Here's how the part is built. I have some questions about the finished solid (model axes, mm). A direction names the side the tool comes from. Coordinates: 2 decimals unless noted, no trailing zeros. Write each loop counter-clockwise with the first axis right and the second up, starting at its lowest first coordinate (ties: lowest second). Pieces come first, ordered by that corner, then holes. Notation, with made-up numbers: (38, 48.5) -> (80, 48.5) arc R21 ccw to (80, 87.5) -> close; hole circle Ø3 at (-4, -35.5). An arc over 180 degrees is marked (long way). Put each result on its own line as item: value.
Autodesk Inventor part; units mm, degrees
ref_plane "YZ Plane" through (0, 0, 0) normal (1, 0, 0) x (0, 1, 0)
ref_plane "XZ Plane" through (0, 0, 0) normal (0, 1, 0) x (-1, 0, 0)
ref_plane "XY Plane" through (0, 0, 0) normal (0, 0, 1) x (1, 0, 0)
sketch "Sketch1" plane through (0, 0, 0) normal (0, 1, 0) x (-1, 0, 0)
  line L0 (0, 0) -> (128, 0)
  line L1 (128, 0) -> (128, 22)
  line L2 (52, 14) -> (52, 8)
  line L3 (52, 8) -> (22, 8)
  line L4 (22, 8) -> (22, 14)
  circle A0 centre (5.5, 18.5) radius 2.25
  circle A1 centre (5.5, 18.5) radius 4.5 construction
  circle A2 centre (25.5, 18.5) radius 2.25
  circle A3 centre (25.5, 18.5) radius 4.5 construction
  line L5 (33, 14) -> (44, 14) construction
  circle A4 centre (38.5, 19.099) radius 7.5 construction
  circle A5 centre (38.5, 19.099) radius 4 construction
  line L6 (33, 23) -> (33, 14)
  line L7 (44, 14) -> (44, 23)
  line L8 (22, 14) -> (33, 14)
  line L9 (44, 14) -> (52, 14)
  line L10 (0, 14) -> (4, 14)
  line L11 (4, 14) -> (4, 8)
  line L12 (4, 8) -> (0, 8)
  line L13 (0, 23) -> (0, 14)
  line L14 (0, 8) -> (0, 0)
  line L15 (11.5, 23) -> (11.5, 29)
  line L16 (13.5, 31) -> (17.5, 31)
  line L17 (19.5, 29) -> (19.5, 23)
  arc A6 (13.5, 31) -> (11.5, 29) centre (13.5, 29) ccw
  arc A7 (19.5, 29) -> (17.5, 31) centre (17.5, 29) ccw
  line L18 (33, 23) -> (19.5, 23)
  line L19 (11.5, 23) -> (0, 23)
  line L20 (50, 23) -> (50, 29)
  line L21 (52, 31) -> (56, 31)
  line L22 (58, 29) -> (58, 23)
  arc A8 (52, 31) -> (50, 29) centre (52, 29) ccw
  arc A9 (58, 29) -> (56, 31) centre (56, 29) ccw
  line L23 (68, 23) -> (58, 23)
  line L24 (50, 23) -> (44, 23)
  line L25 (68, 23) -> (68, 22)
  line L26 (68, 22) -> (128, 22)
  line L27 (19.5, 16.7896) -> (15.5, 14.4802)
  line L28 (15.5, 14.4802) -> (11.5, 16.7896)
  line L29 (11.5, 16.7896) -> (11.5, 21.4084)
  line L30 (11.5, 21.4084) -> (15.5, 23.7178)
  line L31 (15.5, 23.7178) -> (19.5, 21.4084)
  line L32 (19.5, 21.4084) -> (19.5, 16.7896)
  point P0 (15.5, 19.099)
  point P1 (0, 18.5)
  point P2 (15.5, 31)
  point P3 (15.5, 19.099)
  dimension "d0" = 6
  dimension "d1" = 8
  dimension "d3" = 4.5
  dimension "d4" = 9
  dimension "d5" = 4.5
  dimension "d6" = 9
  dimension "d8" = 11
  dimension "d9" = 8
  dimension "d10" = 15
  dimension "d11" = 9
  dimension "d12" = 4
  dimension "d13" = 5.5
  dimension "d14" = 10
  dimension "d15" = 10
  dimension "d16" = 2
  dimension "d17" = 8
  dimension "d18" = 8
  dimension "d19" = 23
  dimension "d20" = 30
  dimension "d21" = 18
  dimension "d23" = 2
  dimension "d24" = 8
  dimension "d25" = 6
  dimension "d26" = 8
  dimension "d27" = 10
  dimension "d29" = 60
  dimension "d30" = 8
extrude "Extrusion1" add sketch "Sketch1" along normal blind 6
sketch "Sketch2" plane through (0, 6, 0) normal (0, 1, 0) x (1, 0, 0)
  line L0 (-128, 0) -> (-128, -22)
  line L1 (-128, -22) -> (-68, -22)
  line L2 (-68, -22) -> (-68, -23)
  line L3 (-120, -22) -> (-112, -22)
  line L4 (-112, -22) -> (-112, -26)
  line L5 (-114, -28) -> (-118, -28)
  line L6 (-120, -26) -> (-120, -22)
  line L7 (-84, -22) -> (-76, -22)
  line L8 (-76, -22) -> (-76, -26)
  line L9 (-78, -28) -> (-82, -28)
  line L10 (-84, -26) -> (-84, -22)
  arc A0 (-84, -26) -> (-82, -28) centre (-82, -26) ccw
  arc A1 (-78, -28) -> (-76, -26) centre (-78, -26) ccw
  arc A2 (-114, -28) -> (-112, -26) centre (-114, -26) ccw
  arc A3 (-120, -26) -> (-118, -28) centre (-118, -26) ccw
  dimension "d33" = 2
  dimension "d34" = 8
  dimension "d35" = 6
  dimension "d36" = 8
  dimension "d37" = 8
  dimension "d38" = 8
extrude "Extrusion2" add sketch "Sketch2" against normal blind 6
sketch "Sketch3" plane through (0, 6, 0) normal (0, 1, 0) x (1, 0, 0)
  line L0 (0, 0) -> (-128, 0)
  line L1 (-112, -26) -> (-112, -22)
  line L2 (-76, -26) -> (-76, -22)
  line L3 (0, -8) -> (0, 0)
  line L4 (-120, 0) -> (-112, 0)
  line L5 (-112, 0) -> (-112, 4)
  line L6 (-114, 6) -> (-118, 6)
  line L7 (-120, 4) -> (-120, 0)
  line L8 (-84, 0) -> (-76, 0)
  line L9 (-76, 0) -> (-76, 4)
  line L10 (-78, 6) -> (-82, 6)
  line L11 (-84, 4) -> (-84, 0)
  line L12 (-63, 0) -> (-55, 0)
  line L13 (-55, 0) -> (-55, 4)
  line L14 (-57, 6) -> (-61, 6)
  line L15 (-63, 4) -> (-63, 0)
  line L16 (-12, 0) -> (-4, 0)
  line L17 (-4, 0) -> (-4, 4)
  line L18 (-6, 6) -> (-10, 6)
  line L19 (-12, 4) -> (-12, 0)
  arc A0 (-118, 6) -> (-120, 4) centre (-118, 4) ccw
  arc A1 (-112, 4) -> (-114, 6) centre (-114, 4) ccw
  arc A2 (-82, 6) -> (-84, 4) centre (-82, 4) ccw
  arc A3 (-76, 4) -> (-78, 6) centre (-78, 4) ccw
  arc A4 (-61, 6) -> (-63, 4) centre (-61, 4) ccw
  arc A5 (-55, 4) -> (-57, 6) centre (-57, 4) ccw
  arc A6 (-10, 6) -> (-12, 4) centre (-10, 4) ccw
  arc A7 (-4, 4) -> (-6, 6) centre (-6, 4) ccw
  dimension "d41" = 2
  dimension "d42" = 6
  dimension "d43" = 8
  dimension "d44" = 8
  dimension "d45" = 8
  dimension "d46" = 8
  dimension "d47" = 4
  dimension "d48" = 43
extrude "Extrusion3" add sketch "Sketch3" against normal blind 6
sketch "Sketch4" plane through (0, 0, 0) normal (0, -1, 0) x (1, 0, 0)
  line L0 (-112, 22) -> (-84, 22)
  line L1 (-128, 0) -> (-128, 22)
  line L2 (-84, 0) -> (-112, 0)
  line L3 (-63, 0) -> (-76, 0)
  line L4 (-4, -4) -> (-4, 0)
  line L5 (-124, 14) -> (-124, 8)
  line L6 (-124, 8) -> (-120, 4)
  line L7 (-120, 4) -> (-76, 4)
  line L8 (-76, 4) -> (-72, 8)
  line L9 (-72, 8) -> (-72, 14)
  line L10 (-72, 14) -> (-76, 18)
  line L11 (-76, 18) -> (-120, 18)
  line L12 (-120, 18) -> (-124, 14)
  line L13 (-68, 22) -> (-68, 0) construction
  dimension "d52" = 45
  dimension "d53" = 4
  dimension "d54" = 4
  dimension "d55" = 4
  dimension "d56" = 4
  dimension "d57" = 4
extrude "Extrusion4" cut sketch "Sketch4" against normal blind 6
properties part number "x_iddler_wall_lower"
Item 1: Imagine slicing it at B-B on x = -25.5. Write out the boundary of the cut face in (y, z), then the cut area to 3 significant figures.
Output:
outline: (0, 0) -> (6, 0) -> (6, 8) -> (0, 8) -> close; (0, 14) -> (6, 14) -> (6, 16.25) -> (0, 16.25) -> close; (0, 20.75) -> (6, 20.75) -> (6, 23) -> (0, 23) -> close
area: 75.0 mm²
Item 2: For P1, Ø3, axis at y = 2.5, z = -1, coming from the -X side; P2, Ø1.8, axis at y = 4, z = 25.5, coming from the -X side; P3, Ø1.8, axis at x = -95.5, y = 2.5, coming from the -Z side; P4, Ø3, axis at x = -2, y = 2, coming from the +Z side, each with a flat end and sliding along its axis, tell me the tip position at first contact or that it passes through.
Output:
P1: stops at x = -128
P2: stops at x = -120
P3: stops at z = 0
P4: stops at z = 23
Item 3: If we mould it in two halves opening along X, with no side actions, what happens to faces 4 (the flat face through (-116, 3, -6)), 5 (the flat face through (-47, 3, 23)), 6 (the flat face through (-4, 3, 11))? For each: released by +X, released by -X, zero draft, split by the parting line, or undercut.
Output:
face 4: zero draft
face 5: undercut
face 6: released by +X
Item 4: Which directions (+Z, -Z, +X, -X, +Y, -Y) give clear straight access to the entire face, cutting with the end or side of a thin tool? Please do faces 1 (the flat face through (-37, 3, 8)), 2 (the flat face through (-33, 3, 19)), 3 (the flat face through (-6, 3, 23)).
Output:
face 1: +Y, -Y
face 2: +Z, +Y, -Y
face 3: +Z, +X, +Y, -Y
Item 5: Please list where these lines run through material, in increasing order: line 1 along Z through (x, y) = (-25.5, 1.95); line 2 along X through (y, z) = (0.55, -1.5); line 3 along Z through (x, y) = (-111, 2.7). Write a range as from..to.
Output:
line 1: z = 0..8, 14..16.25, 20.75..23
line 2: x = -120..-112, -84..-76, -63..-55, -12..-4
line 3: z = 0..4, 18..22
Item 6: Imagine slicing it at C-C on y = 4.3. State how many separate pieces and enclosed holes the cut face has, then the cut area to 3 significant figures.
Output:
separate pieces: 1
enclosed holes: 4
area: 2,200 mm²
Item 7: Imagine slicing it at A-A on z = -2. Write out the boundary of the cut face in (x, y).
Output:
outline: (-120, 0) -> (-112, 0) -> (-112, 6) -> (-120, 6) -> close; (-84, 0) -> (-76, 0) -> (-76, 6) -> (-84, 6) -> close; (-63, 0) -> (-55, 0) -> (-55, 6) -> (-63, 6) -> close; (-12, 0) -> (-4, 0) -> (-4, 6) -> (-12, 6) -> close
